Autodesk Inventor part; units mm, degrees
ref_plane "YZ Plane" through (0, 0, 0) normal (1, 0, 0) x (0, 1, 0)
ref_plane "XZ Plane" through (0, 0, 0) normal (0, 1, 0) x (-1, 0, 0)
ref_plane "XY Plane" through (0, 0, 0) normal (0, 0, 1) x (1, 0, 0)
sketch "Sketch1" plane through (0, 0, 0) normal (0, 0, 1) x (1, 0, 0)
  line L0 (0, 0) -> (0, -31.9527)
  line L1 (13.6569, 19) -> (24, 19)
  line L2 (1.4142, 7.5858) -> (12.2426, 18.4142)
  line L3 (26, 17) -> (26, -10)
  line L4 (26, -10) -> (0, -10)
  line L5 (-13.6569, 19) -> (-24, 19)
  line L6 (-1.4142, 7.5858) -> (-12.2426, 18.4142)
  line L7 (-26, 17) -> (-26, -10)
  line L8 (-26, -10) -> (0, -10)
  line L9 (-26, -5) -> (26, -5)
  arc A0 (-24, 19) -> (-26, 17) centre (-24, 17) ccw
  arc A1 (-12.2426, 18.4142) -> (-13.6569, 19) centre (-13.6569, 17) ccw
  arc A2 (-1.4142, 7.5858) -> (1.4142, 7.5858) centre (0, 9) ccw
  arc A3 (13.6569, 19) -> (12.2426, 18.4142) centre (13.6569, 17) ccw
  arc A4 (26, 17) -> (24, 19) centre (24, 17) ccw
  point P0 (-18, 11.5)
  point P1 (18, 11.5)
  point P2 (12.8284, 19)
  point P3 (26, 19)
  point P4 (-12.8284, 19)
  point P5 (-26, 19)
  dimension "d0" = 36
  dimension "d1" = 18
  dimension "d2" = 135
  dimension "d3" = 19
  dimension "d4" = 11.5
  dimension "d5" = 5
  dimension "d6" = 24
  dimension "d7" = 26
  dimension "d10" = 2
  dimension "d11" = 10
extrude "Extrusion1" add sketch "Sketch1" along normal mid plane 5 contours L9 L7 A0 L5 A1 L6 A2 L2 A3 L1 A4 L3
hole "Hole1" at (-18, 11.5, 0) at (18, 11.5, 0) direction (0, 0, -1) diameter 5.159 end through all both
extrude "Extrusion2" add sketch "Sketch1" along normal mid plane 36 contours L9 L3 L4 L0 | L0 L8 L7 L9
fillet "Fillet1" radius 2 4 edges at (-26, -7.5, 18) (26, -7.5, 18) (-26, -7.5, -18) (26, -7.5, -18)
sketch "Sketch2" plane through (-26, -5, -2.5) normal (0, 1, 0) x (1, 0, 0)
  line L0 (42.418, 8.7532) -> (37.087, 8.7532) construction
  line L1 (42.418, 11.2532) -> (37.087, 11.2532)
  line L2 (37.087, 6.2532) -> (42.418, 6.2532)
  arc A0 (42.418, 6.2532) -> (42.418, 11.2532) centre (42.418, 8.7532) ccw
  arc A1 (37.087, 11.2532) -> (37.087, 6.2532) centre (37.087, 8.7532) ccw
  line L3 (69.9256, -2.5) -> (59.9264, -2.5)
  line L4 (36.6897, -2.5) -> (64.1036, -2.5)
  line L5 (42.418, -13.7532) -> (37.087, -13.7532) construction
  line L6 (42.418, -16.2532) -> (37.087, -16.2532)
  line L7 (37.087, -11.2532) -> (42.418, -11.2532)
  arc A2 (42.418, -16.2532) -> (42.418, -11.2532) centre (42.418, -13.7532) ccw
  arc A3 (37.087, -11.2532) -> (37.087, -16.2532) centre (37.087, -13.7532) ccw
  line L8 (52, 0) -> (0, 0)
  line L9 (26, 0) -> (26, 17.4848)
  line L10 (9.582, 8.7532) -> (14.913, 8.7532) construction
  line L11 (9.582, 11.2532) -> (14.913, 11.2532)
  line L12 (14.913, 6.2532) -> (9.582, 6.2532)
  arc A4 (9.582, 11.2532) -> (9.582, 6.2532) centre (9.582, 8.7532) ccw
  arc A5 (14.913, 6.2532) -> (14.913, 11.2532) centre (14.913, 8.7532) ccw
  line L13 (9.582, -13.7532) -> (14.913, -13.7532) construction
  line L14 (9.582, -16.2532) -> (14.913, -16.2532)
  line L15 (14.913, -11.2532) -> (9.582, -11.2532)
  arc A6 (9.582, -11.2532) -> (9.582, -16.2532) centre (9.582, -13.7532) ccw
  arc A7 (14.913, -16.2532) -> (14.913, -11.2532) centre (14.913, -13.7532) ccw
  point P0 (26, -2.5)
  point P1 (39.7525, 8.7532)
  point P2 (39.7525, -13.7532)
  point P3 (26, -2.5)
  point P4 (26, -2.5)
  point P5 (26, -2.5)
  point P6 (12.2475, 8.7532)
  point P7 (15.3103, -2.5)
  point P8 (12.2475, -13.7532)
  dimension "d24" = 5
extrude "Extrusion3" cut sketch "Sketch2" against normal through all
properties part number "basepart"
Verification items for the finished model (mm, model axes). A direction names the side the tool comes from. Give positions to 0.01 mm unless a question says otherwise; leave off trailing zeros. Loops run counter-clockwise (first coordinate to the right, second up) from the corner with the lowest first, then second, coordinate; pieces in that order, holes last.
1. Cross-section at D-D on x = -10. Record the cut outline in (y, z).
Derived:
outline: (-10, -18) - (-5, -18) - (-5, -13.5) - (-10, -13.5) - close; (-10, -9) - (-5, -9) - (-5, -2.5) - (16.17, -2.5) - (16.17, 2.5) - (-5, 2.5) - (-5, 9) - (-10, 9) - close; (-10, 13.5) - (-5, 13.5) - (-5, 18) - (-10, 18) - close
2. Material ranges on probe 1 along Y at (x, z) = (-18, 0.5); probe 2 along X at (y, z) = (-6, -10); probe 3 along X at (y, z) = (11.5, 0.4), recorded low to high.
Derived:
probe 1: y = -10 to 8.92, 14.08 to 19
probe 2: x = -26 to -18.58, -8.92 to 8.92, 18.58 to 26
probe 3: x = -26 to -20.58, -15.42 to -5.33, 5.33 to 15.42, 20.58 to 26
3. Release check for a two-part mould opening along Z. For faces 1 (the flat face through (0, 5, 2.5)), 2 (the cylindrical face through (19.57, 13.547, -0.035)), 3 (the cylindrical face through (8.588, -7.465, 11.198)), 4 (the cylindrical face through (25.4, -7.54, -17.43)) record: +Z half, -Z half, draft (parallel to the pull), parting line (faces both ways), or undercut.
Derived:
face 1: +Z half
face 2: draft
face 3: undercut
face 4: -Z half
4. Go/stop test with flat-tipped pins: P1, Ø12, axis at y = 0, z = 11, coming from the -X side; P2, Ø4, axis at x = -18, y = 11.5, coming from the +Z side; P3, Ø12, axis at x = -13, y = 3, coming from the -Z side; P4, Ø8, axis at x = -12.5, z = -13.5, coming from the +Y side. Record where each tip stops, or that it passes through.
Derived:
P1: stops at x = -26
P2: passes through
P3: stops at z = -2.5
P4: stops at y = -5
5. Cross-section at C-C on x = 20. Record the cut outline in (y, z), and give its area (3 significant figures).
Derived:
outline: (-10, -18) - (-5, -18) - (-5, -2.5) - (9.87, -2.5) - (9.87, 2.5) - (-5, 2.5) - (-5, 18) - (-10, 18) - close; (13.13, -2.5) - (19, -2.5) - (19, 2.5) - (13.13, 2.5) - close
area: 284 mm2
6. Cross-section at A-A on y = -5.75. Record the cut outline in (x, z).
Derived:
outline: (-26, -16) arc R2 ccw to (-24, -18) - (24, -18) arc R2 ccw to (26, -16) - (26, 16) arc R2 ccw to (24, 18) - (-24, 18) arc R2 ccw to (-26, 16) - close; hole (-16.42, -13.75) - (-11.09, -13.75) arc R2.5 ccw to (-11.09, -8.75) - (-16.42, -8.75) arc R2.5 ccw to start; hole (-16.42, 8.75) - (-11.09, 8.75) arc R2.5 ccw to (-11.09, 13.75) - (-16.42, 13.75) arc R2.5 ccw to start; hole (11.09, -13.75) - (16.42, -13.75) arc R2.5 ccw to (16.42, -8.75) - (11.09, -8.75) arc R2.5 ccw to start; hole (11.09, 8.75) - (16.42, 8.75) arc R2.5 ccw to (16.42, 13.75) - (11.09, 13.75) arc R2.5 ccw to start
7. Tool access check on faces 5 (the flat face through (26, 0, 0)), 6 (the flat face through (0, -5, 10)), 7 (the flat face through (0, 5, -2.5)), 8 (the cylindrical face through (-18.917, -7.465, 11.198)). Record the directions out of +Z, -Z, +X, -X, +Y, -Y that give a thin tool (end or side, any length) a straight path to the whole face; none if there is none.
Derived:
face 5: +Z, -Z, +X, +Y, -Y
face 6: +Z, +X, -X, +Y
face 7: -Z, +X, -X, +Y
face 8: +Y, -Y
8. Cross-section at B-B on z = 10. Record the cut outline in (x, y), and give its area (3 significant figures).
Derived:
outline: (-26, -10) - (-18.58, -10) - (-18.58, -5) - (-26, -5) - close; (-8.92, -10) - (8.92, -10) - (8.92, -5) - (-8.92, -5) - close; (18.58, -10) - (26, -10) - (26, -5) - (18.58, -5) - close
area: 163 mm2
